```python
from build123d import *

# Parameters (mm, degrees)
SKETCH006_W     = 95
SKETCH006_H     = 27
PAD003_DEPTH    = 2
SKETCH007_R     = 1.3
POCKET003_DEPTH = 2
FILLET003_R     = 3
SKETCH008_R     = 1.75
SKETCH008_R_2   = 2.7
POCKET004_DEPTH = 2
SKETCH009_W     = 15.7
SKETCH009_H     = 16.2
SKETCH009_W_2   = 16.4
SKETCH009_H_2   = 13.9
POCKET005_DEPTH = 2


with BuildPart() as part:
    # Sketch006 → Pad003 (new body)
    with BuildSketch(Plane.XY):
        Rectangle(SKETCH006_W, SKETCH006_H)
    extrude(amount=PAD003_DEPTH)

    # Sketch007 (on Face6 of Pad003) → Pocket003 (cut)
    with BuildSketch(Plane.XY.offset(2)):
        with Locations((-44.5, 10.5)):
            Circle(SKETCH007_R)
        with Locations((44.5, 10.5)):
            Circle(SKETCH007_R)
        with Locations((44.5, -10.5)):
            Circle(SKETCH007_R)
        with Locations((-44.5, -10.5)):
            Circle(SKETCH007_R)
    extrude(amount=-POCKET003_DEPTH, mode=Mode.SUBTRACT)

    # Fillet003
    fillet003_edges = [part.edges().sort_by_distance(p)[0] for p in [
        (-47.5, -13.5, 1),
        (47.5, -13.5, 1),
        (47.5, 13.5, 1),
        (-47.5, 13.5, 1),
    ]]
    fillet(fillet003_edges, radius=FILLET003_R)

    # Sketch008 (on Face5 of Fillet003) → Pocket004 (cut)
    with BuildSketch(Plane.XY.offset(2)):
        with Locations((-34.4, -0.3)):
            Circle(SKETCH008_R)
        with Locations((-24.1, 0.3)):
            Circle(SKETCH008_R_2)
    extrude(amount=-POCKET004_DEPTH, mode=Mode.SUBTRACT)

    # Sketch009 (on Face5 of Pocket004) → Pocket005 (cut)
    with BuildSketch(Plane.XY.offset(2)):
        with Locations((-6.45, -1.7)):
            Rectangle(SKETCH009_W, SKETCH009_H)
        with Locations((11.85, -1.7)):
            Rectangle(SKETCH009_W, SKETCH009_H)
        with Locations((30.2, -0.55)):
            Rectangle(SKETCH009_W_2, SKETCH009_H_2)
    extrude(amount=-POCKET005_DEPTH, mode=Mode.SUBTRACT)


with BuildPart() as part_1:
    # Body002 placement: moved
    add(part.part.moved(Location((0, -1.2, 135.4))))


solid = part_1.part
```
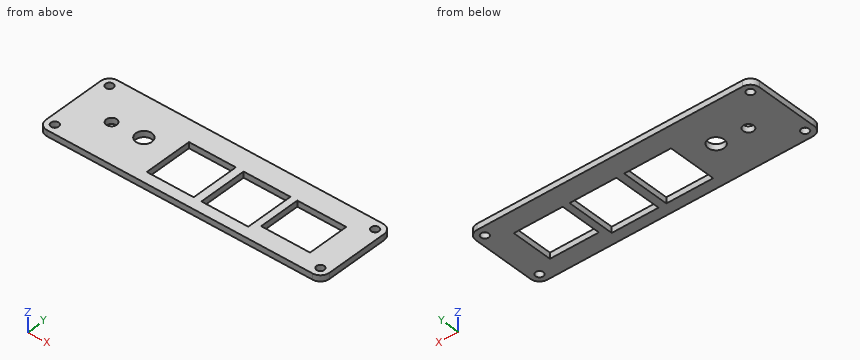
Verification items for the finished model (mm, model axes). Coordinates: 2 decimals unless noted, no trailing zeros. Write each loop counter-clockwise with the first axis right and the second up, starting at its lowest first coordinate (ties: lowest second). Pieces come first, ordered by that corner, then holes. Notation, with made-up numbers: M 88,84 L 111,84 A18 ccw 111,94 Z; hole C 54.5,29 d4. An arc over 180 degrees is marked long. Answer as a JSON object with one key per item and string values. Group by question number.
(1) Cross-section at A-A, the plane x = -4. Record the cut outline in (y, z).
(2) Cross-section at B-B, the plane y = -7. Record the cut outline in (x, z), and give its area (3 significant figures).
(3) Gauge pin test, flat end, axial feed: pin 1 (8.5 mm diameter, centred on x = -24.1, y = -0.9, fed in from +Z). Record the tip position at first contact, or that the pin passes through.
(4) Material ranges on line 1 (X direction, y = -4.75, z = 136.65); line 2 (Y direction, x = 44.5, z = 136.05); line 3 (X direction, y = -9.5, z = 136.6), recorded low to high.
(5) Cross-section at C-C, the plane z = 136.75. State how many separate pieces and enclosed holes the cut face has, and give its area (3 significant figures).
(6) Cross-section at D-D, the plane x = -24.1. Record the cut outline in (y, z), and give its area (3 significant figures).
Reply:
{
 "1": {"outline": "M -14.7,135.4 L -11,135.4 L -11,137.4 L -14.7,137.4 Z; M 5.2,135.4 L 12.3,135.4 L 12.3,137.4 L 5.2,137.4 Z"},
 "2": {"outline": "M -47.5,135.4 L -14.3,135.4 L -14.3,137.4 L -47.5,137.4 Z; M 1.4,135.4 L 4,135.4 L 4,137.4 L 1.4,137.4 Z; M 19.7,135.4 L 22,135.4 L 22,137.4 L 19.7,137.4 Z; M 38.4,135.4 L 47.5,135.4 L 47.5,137.4 L 38.4,137.4 Z", "area": "94.4 mm²"},
 "3": {"pin 1": "z = 137.4"},
 "4": {"line 1": "-47.5 to -14.3, 1.4 to 4, 19.7 to 22, 38.4 to 47.5", "line 2": "-14.7 to -13, -10.4 to 8, 10.6 to 12.3", "line 3": "-47.5 to -14.3, 1.4 to 4, 19.7 to 47.5"},
 "5": {"separate pieces": "1", "enclosed holes": "9", "area": "1,770 mm²"},
 "6": {"outline": "M -14.7,135.4 L -3.6,135.4 L -3.6,137.4 L -14.7,137.4 Z; M 1.8,135.4 L 12.3,135.4 L 12.3,137.4 L 1.8,137.4 Z", "area": "43.2 mm²"}
}
